from build123d import *

# Parameters (mm, degrees)
SKETCH_1_W             = 20
SKETCH_1_H             = 20
EXTRUDE_1_DEPTH        = 690
SKETCH_2_W             = 32
SKETCH_2_H             = 32
EXTRUDE_2_DEPTH        = 50
SKETCH_3_W             = 30
SKETCH_3_H             = 30
CUT_EXTRUDE_1_DEPTH    = 46
SKETCH_4_W             = 300
SKETCH_4_H             = 5
EXTRUDE_3_DEPTH        = 20
PATTERN_LINEAR_1_COUNT = 2
PATTERN_LINEAR_1_PITCH = 57


with BuildPart() as part:
    # 草图1 → 凸台-拉伸1 (new body)
    with BuildSketch(Plane.XY):
        Rectangle(SKETCH_1_W, SKETCH_1_H)
    extrude(amount=EXTRUDE_1_DEPTH)

    # 草图2 → 凸台-拉伸2 (add)
    with BuildSketch(Plane(origin=(0, 0, 0), x_dir=(-1, 0, 0), z_dir=(0, 0, -1))):
        Rectangle(SKETCH_2_W, SKETCH_2_H)
    extrude(amount=EXTRUDE_2_DEPTH)

    # 草图3 → 切除-拉伸1 (cut)
    with BuildSketch(Plane(origin=(0, 0, -50), x_dir=(-1, 0, 0), z_dir=(0, 0, -1))):
        Rectangle(SKETCH_3_W, SKETCH_3_H)
    extrude(amount=-CUT_EXTRUDE_1_DEPTH, mode=Mode.SUBTRACT)

    # 草图4 → 凸台-拉伸3 (add)
    with BuildSketch(Plane(origin=(0, 10, 0), x_dir=(1, 0, 0), z_dir=(0, 1, 0))):
        with Locations((0, 47.5)):
            Rectangle(SKETCH_4_W, SKETCH_4_H)
    extrude_3 = extrude(amount=-EXTRUDE_3_DEPTH)

    # 阵列(线性)1: 凸台-拉伸3 ×2
    with Locations(*[(0, 0, i * PATTERN_LINEAR_1_PITCH) for i in range(1, PATTERN_LINEAR_1_COUNT)]):
        add(extrude_3)


solid = part.part
Work out the finished part from the listing and answer in its coordinate system (mm). A direction names the side the tool comes from. Coordinates: 2 decimals unless noted, no trailing zeros. Loops run counter-clockwise (first coordinate to the right, second up) from the corner with the lowest first, then second, coordinate; pieces in that order, holes last. Notation, with made-up numbers: (10.5, -38) -> (27.5, -38) arc R16 cw to (27.5, -18) -> close; hole circle Ø1 at (64, 25). An arc over 180 degrees is marked (long way). Write each question's results on one line, items separated by ' | '. Start each with the question number.
1) Find section A-A on y = 0.5. Determine the outline of the cut face in (x, z), then the cut area to 3 significant figures.
2) Consider line 1 along Z through (x, y) = (111.5, 6); line 2 along X through (y, z) = (-5, -2); line 3 along X through (y, z) = (4, 93.5). Determine where each line is inside the solid, lowest interval first.
3) Find section B-B on x = -28. Determine the outline of the cut face in (y, z).
4) The mould has two halves that part along Y. Classify faces 5 (the flat face through (0, 0, -45)), 6 (the flat face through (-1, -10, 190)), 7 (the flat face through (10, 0, 346)): pulls with the +Y half, pulls with the -Y half, needs draft (parallel to the pull), parting line crosses it, or undercut.
5) Flat-ended cylindrical pins translate along their axes: P1, Ø15, axis at y = 2, z = -24.5, coming from the +X side; P2, Ø16, axis at x = -51.5, y = 1.5, coming from the +Z side; P3, Ø8, axis at y = 8.5, z = 562, coming from the +X side. Find the tip coordinate at first contact, or state that the pin passes through.
6) Find section C-C on z = 435.5. Determine the outline of the cut face in (x, y), then the cut area to 3 significant figures.
7) For faces 1 (the flat face through (-81, 0, 7)), 2 (the flat face through (79, 0, 7)), 3 (the flat face through (0, -15, -27)), 4 (the flat face through (0, 0, -4)), determine the directions among +Z, -Z, +X, -X, +Y, -Y from which every point of the face is accessible in a straight line to the end or side of a thin tool.
Response values:
1) outline: (-150, -50) -> (150, -50) -> (150, -45) -> (16, -45) -> (16, 0) -> (10, 0) -> (10, 7) -> (150, 7) -> (150, 12) -> (10, 12) -> (10, 690) -> (-10, 690) -> (-10, 12) -> (-150, 12) -> (-150, 7) -> (-10, 7) -> (-10, 0) -> (-16, 0) -> (-16, -45) -> (-150, -45) -> close; hole (-15, -45) -> (15, -45) -> (15, -4) -> (-15, -4) -> close | area: 16,900 mm^2
2) line 1: z = -50 to -45, 7 to 12 | line 2: x = -16 to 16 | line 3: x = -10 to 10
3) outline: (-10, -50) -> (10, -50) -> (10, -45) -> (-10, -45) -> close; (-10, 7) -> (10, 7) -> (10, 12) -> (-10, 12) -> close
4) face 5: undercut | face 6: pulls with the -Y half | face 7: needs draft
5) P1: stops at x = 16 | P2: stops at z = 12 | P3: stops at x = 10
6) outline: (-10, -10) -> (10, -10) -> (10, 10) -> (-10, 10) -> close | area: 400 mm^2
7) face 1: -X, +Y, -Y | face 2: +X, +Y, -Y | face 3: -Z | face 4: none
